Part model, mm, in its own coordinate system. Face numbers are marked on the shaded views. Give positions to 0.01 mm unless a question says otherwise; leave off trailing zeros. Write each loop counter-clockwise with the first axis right and the second up, starting at its lowest first coordinate (ties: lowest second). Pieces come first, ordered by that corner, then holes. Notation, with made-up numbers: M -20,60 L 10,60 A29 cw 10,94 Z; hole C -8,26 d7. An arc over 180 degrees is marked long. Answer as CSV lines item,"result". Start each with the question number.
Item 1: Pin check, flat tips, straight feed: pin 1 (3 mm diameter, centred on x = 8, y = 6, fed in from +Z); pin 2 (1 mm diameter, centred on y = 4, z = -5, fed in from -X); pin 3 (14 mm diameter, centred on x = 0, z = 0, fed in from +Y); pin 4 (2 mm diameter, centred on y = 2.5, z = -10, fed in from -X). Stop position of each tip, or through.
Item 2: Two-plate mould, pull along Y, no slides. Class the marked faces 1 and 2: +Y half, -Y half, draft (parallel to the pull), parting line (faces both ways), or undercut.
Item 3: Wall check: L1, parallel to X at y = 6.55, z = 0; L2, parallel to X at y = 2.4, z = 0; L3, parallel to Y at x = 8.5, z = -14. Give the ranges that are in metal, low to high. Write a range as from..to.
Item 4: Band-saw the part on B-B, the plane y = 5.75. List the corners of the cut face in (x, z).
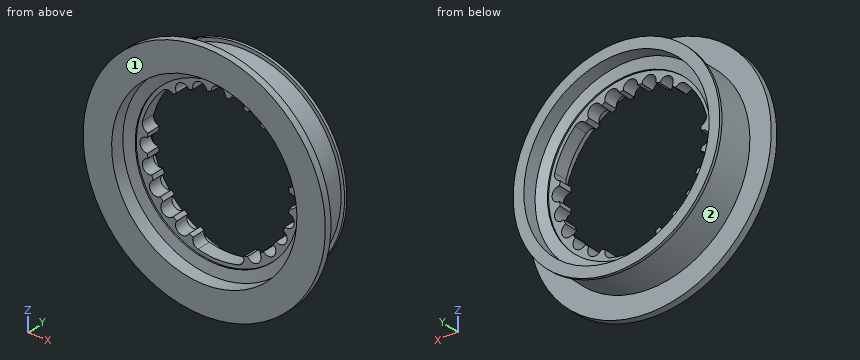
from build123d import *

# Parameters (mm, degrees)
SKETCH_1_R          = 17
EXTRUDE_1_DEPTH     = 1
SKETCH_2_R          = 14
EXTRUDE_2_DEPTH     = 5.6
SKETCH_3_R          = 14.5
EXTRUDE_3_DEPTH     = 0.4
CUT_EXTRUDE_1_REACH = 26.459


with BuildPart() as part:
    # 草图1 → 凸台-拉伸1 (new body)
    with BuildSketch(Plane(origin=(0, 0, 0), x_dir=(1, 0, 0), z_dir=(0, 1, 0))):
        with Locations(Location((0, 0, 0), (0, 0, 270))):
            Circle(SKETCH_1_R)
    extrude(amount=EXTRUDE_1_DEPTH)

    # 草图2 → 凸台-拉伸2 (add)
    with BuildSketch(Plane(origin=(0, 1, 0), x_dir=(1, 0, 0), z_dir=(0, 1, 0))):
        with Locations(Location((0, 0, 0), (0, 0, 270))):
            Circle(SKETCH_2_R)
    extrude(amount=EXTRUDE_2_DEPTH)

    # 草图3 → 凸台-拉伸3 (add)
    with BuildSketch(Plane(origin=(0, 6.6, 0), x_dir=(1, 0, 0), z_dir=(0, 1, 0))):
        with Locations(Location((0, 0, 0), (0, 0, 270))):
            Circle(SKETCH_3_R)
    extrude(amount=EXTRUDE_3_DEPTH)

    # 草图4 → 切除-旋转1 (revolve, cut)
    with BuildSketch(Plane(origin=(0, 0, 0), x_dir=(0, 0, -1), z_dir=(1, 0, 0))):
        Polygon((0, 0), (13, 0), (13, 2), (11.5, 2.3), (11.5, 2.5), (0, 2.5), align=None)
        Polygon((11.5, 4.7), (11.5, 4.5), (0, 4.5), (0, 7), (13, 7), (13, 5), align=None)
    revolve(axis=Axis((0, 4.5, 0), (0, 1, 0)), mode=Mode.SUBTRACT)

    # 草图5 → 切除-拉伸1 (cut, up to next)
    with BuildSketch(Plane(origin=(0, 4.5, 0), x_dir=(1, 0, 0), z_dir=(0, 1, 0)), mode=Mode.PRIVATE) as cut_extrude_1_sk1:
        with BuildLine():
            ThreePointArc((3.539967162, 9.352466653), (3.466448921, 10.137444482), (2.847009496, 10.625184089))
            ThreePointArc((2.847009496, 10.625184089), (0, 11), (-2.847009496, 10.625184089))
            ThreePointArc((-2.847009496, 10.625184089), (-3.466448921, 10.137444482), (-3.539967162, 9.352466653))
            ThreePointArc((-3.539967162, 9.352466653), (-3.826834324, 9.238795325), (-4.110057805, 9.116327377))
            ThreePointArc((-4.110057805, 9.116327377), (-5.5, 9.526279442), (-5.839942195, 8.117578159))
            ThreePointArc((-5.839942195, 8.117578159), (-6.08761429, 7.933533403), (-6.329490128, 7.741934817))
            ThreePointArc((-6.329490128, 7.741934817), (-7.778174593, 7.778174593), (-7.741934817, 6.329490128))
            ThreePointArc((-7.741934817, 6.329490128), (-7.933533403, 6.08761429), (-8.117578159, 5.839942195))
            ThreePointArc((-8.117578159, 5.839942195), (-9.526279442, 5.5), (-9.116327377, 4.110057805))
            ThreePointArc((-9.116327377, 4.110057805), (-9.238795325, 3.826834324), (-9.352466653, 3.539967162))
            ThreePointArc((-9.352466653, 3.539967162), (-10.625184089, 2.847009496), (-9.86945729, 1.610531835))
            ThreePointArc((-9.86945729, 1.610531835), (-9.914448614, 1.305261922), (-9.95, 0.998749218))
            ThreePointArc((-9.95, 0.998749218), (-11, 0), (-9.95, -0.998749218))
            ThreePointArc((-9.95, -0.998749218), (-9.914448614, -1.305261922), (-9.86945729, -1.610531835))
            ThreePointArc((-9.86945729, -1.610531835), (-10.512508911, -2.066689415), (-10.625184089, -2.847009496))
            ThreePointArc((-10.625184089, -2.847009496), (-9.526279442, -5.5), (-7.778174593, -7.778174593))
            ThreePointArc((-7.778174593, -7.778174593), (-7.046059991, -8.070755067), (-6.329490128, -7.741934817))
            ThreePointArc((-6.329490128, -7.741934817), (-6.08761429, -7.933533403), (-5.839942195, -8.117578159))
            ThreePointArc((-5.839942195, -8.117578159), (-5.5, -9.526279442), (-4.110057805, -9.116327377))
            ThreePointArc((-4.110057805, -9.116327377), (-3.826834324, -9.238795325), (-3.539967162, -9.352466653))
            ThreePointArc((-3.539967162, -9.352466653), (-2.847009496, -10.625184089), (-1.610531835, -9.86945729))
            ThreePointArc((-1.610531835, -9.86945729), (-1.305261922, -9.914448614), (-0.998749218, -9.95))
            ThreePointArc((-0.998749218, -9.95), (0, -11), (0.998749218, -9.95))
            ThreePointArc((0.998749218, -9.95), (1.305261922, -9.914448614), (1.610531835, -9.86945729))
            ThreePointArc((1.610531835, -9.86945729), (2.847009496, -10.625184089), (3.539967162, -9.352466653))
            ThreePointArc((3.539967162, -9.352466653), (3.826834324, -9.238795325), (4.110057805, -9.116327377))
            ThreePointArc((4.110057805, -9.116327377), (5.5, -9.526279442), (5.839942195, -8.117578159))
            ThreePointArc((5.839942195, -8.117578159), (6.08761429, -7.933533403), (6.329490128, -7.741934817))
            ThreePointArc((6.329490128, -7.741934817), (7.046059991, -8.070755067), (7.778174593, -7.778174593))
            ThreePointArc((7.778174593, -7.778174593), (9.526279442, -5.5), (10.625184089, -2.847009496))
            ThreePointArc((10.625184089, -2.847009496), (10.512508911, -2.066689415), (9.86945729, -1.610531835))
            ThreePointArc((9.86945729, -1.610531835), (9.914448614, -1.305261922), (9.95, -0.998749218))
            ThreePointArc((9.95, -0.998749218), (11, 0), (9.95, 0.998749218))
            ThreePointArc((9.95, 0.998749218), (9.914448614, 1.305261922), (9.86945729, 1.610531835))
            ThreePointArc((9.86945729, 1.610531835), (10.625184089, 2.847009496), (9.352466653, 3.539967162))
            ThreePointArc((9.352466653, 3.539967162), (9.238795325, 3.826834324), (9.116327377, 4.110057805))
            ThreePointArc((9.116327377, 4.110057805), (9.526279442, 5.5), (8.117578159, 5.839942195))
            ThreePointArc((8.117578159, 5.839942195), (7.933533403, 6.08761429), (7.741934817, 6.329490128))
            ThreePointArc((7.741934817, 6.329490128), (7.778174593, 7.778174593), (6.329490128, 7.741934817))
            ThreePointArc((6.329490128, 7.741934817), (6.08761429, 7.933533403), (5.839942195, 8.117578159))
            ThreePointArc((5.839942195, 8.117578159), (5.5, 9.526279442), (4.110057805, 9.116327377))
            ThreePointArc((4.110057805, 9.116327377), (3.826834324, 9.238795325), (3.539967162, 9.352466653))
        make_face()
    cut_extrude_1_tool1 = extrude(cut_extrude_1_sk1.sketch, amount=-CUT_EXTRUDE_1_REACH, mode=Mode.PRIVATE) & part.part
    add(cut_extrude_1_tool1.solids().sort_by_distance((0, 4.5, 0))[0], mode=Mode.SUBTRACT)


solid = part.part
Output:
1,pin 1,"z = 12.9"
1,pin 2,"x = -13.26"
1,pin 3,"through"
1,pin 4,"x = -10.72"
2,face 1,"-Y half"
2,face 2,"undercut"
3,L1,"-14..-13, 13..14"
3,L2,"-14..-11.5, 11.5..14"
3,L3,"0..1"
4,outline,"C 0,0 d28; hole C 0,0 d26"
